Part model, mm, in its own coordinate system. Face numbers are marked on the shaded views. A direction names the side the tool comes from. Round coordinates to 2 decimals unless told otherwise and drop trailing zeros. Loops run counter-clockwise (first coordinate to the right, second up) from the corner with the lowest first, then second, coordinate; pieces in that order, holes last. Notation, with made-up numbers: (75, 27) -> (91, 27) arc R26 ccw to (91, 49) -> close; hole circle Ø3 at (52, -38). An arc over 180 degrees is marked (long way). Answer as CSV lines item,"result".
from build123d import *

# Parameters (mm, degrees)
SKETCH1_R                                           = 60.625
SKETCH1_R_2                                         = 45
BOSS_EXTRUDE1_DEPTH                                 = 4
SKETCH2_R                                           = 49
SKETCH2_R_2                                         = 45
BOSS_EXTRUDE2_DEPTH                                 = 52
SKETCH3_W                                           = 13.25
SKETCH3_H                                           = 8
SKETCH3_W_2                                         = 8
SKETCH3_H_2                                         = 38
BOSS_EXTRUDE3_DEPTH                                 = 13
SKETCH4_W                                           = 24
SKETCH4_H                                           = 10
CUT_EXTRUDE1_DEPTH                                  = 26
SKETCH5_R                                           = 5
CUT_EXTRUDE2_DEPTH                                  = 74
SKETCH6_R                                           = 1.3
CUT_EXTRUDE3_DEPTH                                  = 7.2
BOSS_EXTRUDE4_DEPTH                                 = 4
CSK_FOR_M3_COUNTERSUNK_FLAT_HEAD_SCREW1_D           = 3.4
CSK_FOR_M3_COUNTERSUNK_FLAT_HEAD_SCREW1_DEPTH       = 4
CSK_FOR_M3_COUNTERSUNK_FLAT_HEAD_SCREW1_CSINK_D     = 6.3
CSK_FOR_M3_COUNTERSUNK_FLAT_HEAD_SCREW1_CSINK_ANGLE = 90
CSK_FOR_M3_COUNTERSUNK_FLAT_HEAD_SCREW1_TIP         = 1.021463052
FILLET1_R                                           = 1


with BuildPart() as part:
    # Sketch1 → Boss-Extrude1 (new body)
    with BuildSketch(Plane.XY):
        Circle(SKETCH1_R)
        Circle(SKETCH1_R_2, mode=Mode.SUBTRACT)
    extrude(amount=BOSS_EXTRUDE1_DEPTH)

    # Sketch2 → Boss-Extrude2 (add)
    with BuildSketch(Plane.XY.offset(4)):
        with Locations(Location((0, 0, 0), (0, 0, 180))):
            Circle(SKETCH2_R)
        Circle(SKETCH2_R_2, mode=Mode.SUBTRACT)
    extrude(amount=BOSS_EXTRUDE2_DEPTH)

    # Sketch3 → Boss-Extrude3 (add, symmetric)
    with BuildSketch(Plane(origin=(0, 0, 0), x_dir=(1, 0, 0), z_dir=(0, 1, 0))):
        with Locations((-38.375, -34)):
            Rectangle(SKETCH3_W, SKETCH3_H)
        Polygon((-45, -16.75), (-45, -30), (-31.75, -30), align=None)
        with Locations((15.25, -19)):
            Rectangle(SKETCH3_W_2, SKETCH3_H_2)
    extrude(amount=BOSS_EXTRUDE3_DEPTH, both=True)


with BuildPart() as boss_extrude3_piece_1:
    # of the separate pieces the step leaves, piece 1, a body of its own (boss_extrude3_pieces)
    add(part.part.solids().sort_by_distance((60.625, 0, 0))[0])

    # Sketch5 → Cut-Extrude2 (cut)
    with BuildSketch(Plane.ZY.offset(-11.25)):
        with Locations((14, 0)):
            Circle(SKETCH5_R)
    extrude(amount=-CUT_EXTRUDE2_DEPTH, mode=Mode.SUBTRACT)


with BuildPart() as boss_extrude3_piece_2:
    # of the separate pieces the step leaves, piece 2, a body of its own (boss_extrude3_pieces)
    add(part.part.solids().sort_by_distance((19.25, -13, 0))[0])

    # Sketch4 → Cut-Extrude1 (cut)
    with BuildSketch(Plane.ZY.offset(-11.25)):
        with Locations((17, 0)):
            Rectangle(SKETCH4_W, SKETCH4_H)
    extrude(amount=-CUT_EXTRUDE1_DEPTH, mode=Mode.SUBTRACT)


with BuildPart() as cut_extrude3_tool:
    # Sketch6 → Cut-Extrude3 (new body)
    with BuildSketch(Plane.XY.offset(38)):
        with Locations((-34.25, 5)):
            Circle(SKETCH6_R)
        with Locations((-34.25, -5)):
            Circle(SKETCH6_R)
        with Locations((14.281113412, 5)):
            Circle(SKETCH6_R)
        with Locations((14.281113412, -5)):
            Circle(SKETCH6_R)
    extrude(amount=-CUT_EXTRUDE3_DEPTH)


with BuildPart() as boss_extrude3_piece_1_1:
    add(boss_extrude3_piece_1.part)

    # Cut-Extrude3: cut by cut_extrude3_tool
    add(cut_extrude3_tool.part, mode=Mode.SUBTRACT)



with BuildPart() as boss_extrude3_piece_2_1:
    add(boss_extrude3_piece_2.part)

    # Cut-Extrude3: cut by cut_extrude3_tool
    add(cut_extrude3_tool.part, mode=Mode.SUBTRACT)


with BuildPart() as boss_extrude3_piece_1_2:
    add(boss_extrude3_piece_1_1.part)

    add(boss_extrude3_piece_2_1.part)  # Boss-Extrude4 merges Boss-Extrude3 piece 2
    # Sketch8 → Boss-Extrude4 (add)
    with BuildSketch(Plane(origin=(0, 0, 0), x_dir=(-1, 0, 0), z_dir=(0, 0, -1))):
        with BuildLine():
            Line((-11.25, 13), (-11.25, -13))
            Line((-11.25, -13), (-25.249838503, -37.248431585))
            ThreePointArc((-25.249838503, -37.248431585), (-45, 0), (-25.249838503, 37.248431585))
            Line((-25.249838503, 37.248431585), (-11.25, 13))
        make_face()
        with BuildLine():
            Line((-24.25, -19.516660498), (-27.361802413, -24.906460381))
            ThreePointArc((-27.361802413, -24.906460381), (-37, 0), (-27.361802413, 24.906460381))
            Line((-27.361802413, 24.906460381), (-24.25, 19.516660498))
            Line((-24.25, 19.516660498), (-24.25, -19.516660498))
        make_face(mode=Mode.SUBTRACT)
    extrude(amount=-BOSS_EXTRUDE4_DEPTH)

    # CSK for M3 Countersunk Flat Head Screw1
    with Locations(Plane.XY.offset(4)):
        with Locations((-42, -35), (42, -35), (42, 35), (-42, 35)):
            CounterSinkHole(CSK_FOR_M3_COUNTERSUNK_FLAT_HEAD_SCREW1_D / 2, CSK_FOR_M3_COUNTERSUNK_FLAT_HEAD_SCREW1_CSINK_D / 2, depth=CSK_FOR_M3_COUNTERSUNK_FLAT_HEAD_SCREW1_DEPTH, counter_sink_angle=CSK_FOR_M3_COUNTERSUNK_FLAT_HEAD_SCREW1_CSINK_ANGLE)
            with Locations((0, 0, -(CSK_FOR_M3_COUNTERSUNK_FLAT_HEAD_SCREW1_DEPTH + CSK_FOR_M3_COUNTERSUNK_FLAT_HEAD_SCREW1_TIP / 2))):  # 118° drill point
                Cone(0, CSK_FOR_M3_COUNTERSUNK_FLAT_HEAD_SCREW1_D / 2, CSK_FOR_M3_COUNTERSUNK_FLAT_HEAD_SCREW1_TIP, mode=Mode.SUBTRACT)

    # Fillet1
    fillet1_edges = [boss_extrude3_piece_1_2.edges().sort_by_distance(p)[0] for p in [
        (49, 0, 4),
    ]]
    fillet(fillet1_edges, radius=FILLET1_R)


solid = boss_extrude3_piece_1_2.part
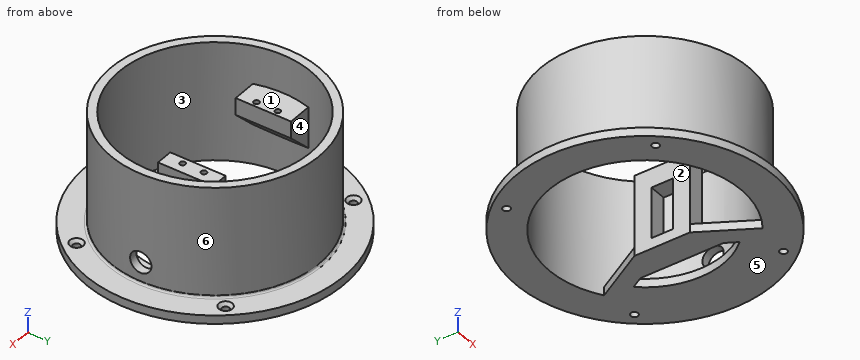
Q1. Saw through at A-A, the plane z = 7.5. Write the cut outline in (x, y), then the cut area to 3 significant figures.
Geometry results:
outline,"circle Ø98 at (0, 0); (11.25, -13) -> (19.25, -13) -> (19.25, -5) -> (11.25, -5) -> close; (11.25, 5) -> (19.25, 5) -> (19.25, 13) -> (11.25, 13) -> close; hole circle Ø90 at (0, 0)"
area,"1,310 mm2"
Q2. Drop flat-ended pins along their axis: P1, Ø9, axis at x = 14.5, y = 5.5, coming from the +Z side; P2, Ø1, axis at y = 44, z = 39, coming from the -X side; P3, Ø6, axis at y = 16.5, z = 22, coming from the -X side; P4, Ø9, axis at x = 14.5, y = 0, coming from the -Z side. Give the stop position or say it passes through.
Geometry results:
P1,"z = 38"
P2,"x = -22.56"
P3,"x = -47.1"
P4,"z = 0"
Q3. Which spindle directions (+Z, -Z, +X, -X, +Y, -Y) get a long thin tool onto all of the face, cutting with end or side? Do the marked faces 1 and 2. Say none if no direction does.
Geometry results:
face 1,"+Z"
face 2,"+Z, -Z"
Q4. Two-plate mould, pull along X, no slides. Class the marked faces 3, 4, 5 and 6: pulls with the +X half, pulls with the -X half, needs draft (parallel to the pull), parting line crosses it, or undercut.
Geometry results:
face 3,"undercut"
face 4,"undercut"
face 5,"needs draft"
face 6,"parting line crosses it"
Q5. Drill centre lines: line 1 along Y through (x, z) = (1, 20.5); line 2 along Y through (x, z) = (-39, 33); line 3 along Z through (x, y) = (-1.5, 53). Where is each one in solid material? Low to high.
Geometry results:
line 1,"-48.99 to -44.99, 44.99 to 48.99"
line 2,"-29.66 to -22.45, -13 to 13, 22.45 to 29.66"
line 3,"0 to 4"
Q6. Saw through at D-D, the plane y = 15. Give the number of separate pieces and of enclosed holes in the cut face, then the cut area to 3 significant figures.
Geometry results:
separate pieces,"3"
enclosed holes,"0"
area,"652 mm2"
Q7. Saw through at C-C, the plane z = 45. Write the cut outline in (x, y), then the cut area to 3 significant figures.
Geometry results:
outline,"circle Ø98 at (0, 0); hole circle Ø90 at (0, 0)"
area,"1,180 mm2"
Q8. Saw through at B-B, the plane x = 0. Write the cut outline in (y, z) (3 decimals), then the cut area to 3 significant figures.
Geometry results:
outline,"(-60.625, 0) -> (-45, 0) -> (-45, 56) -> (-49, 56) -> (-49, 5) arc R1 cw to (-50, 4) -> (-60.625, 4) -> close; (45, 0) -> (60.625, 0) -> (60.625, 4) -> (50, 4) arc R1 cw to (49, 5) -> (49, 56) -> (45, 56) -> close"
area,"541 mm2"
